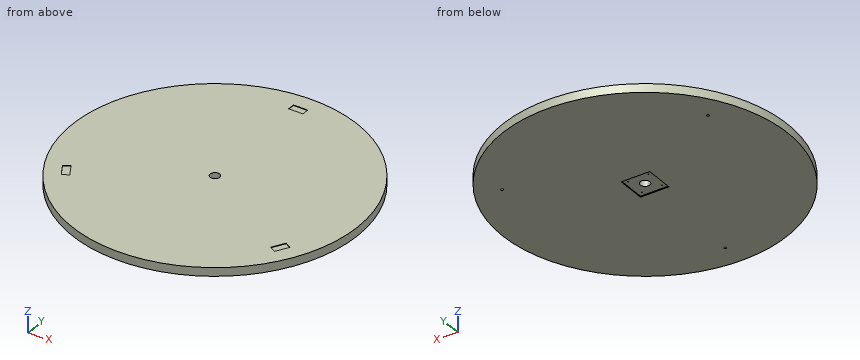
```python
from build123d import *

# Parameters (mm, degrees)
F0_R            = 300
F0_R_2          = 10
F1_DEPTH        = 18
F2_R            = 2.5
F3_DEPTH        = 10
F3_COPIES_COUNT = 3
F4_W            = 60
F4_H            = 60
F5_DEPTH        = 2
F6_R            = 1
F7_DEPTH        = 5
F7_COPIES_COUNT = 4
F8_W            = 30
F8_H            = 15
F9_DEPTH        = 1
F9_COPIES_COUNT = 3


# Not quite as in the source:
# - a pattern or mirror of a feature is missing from the dataset's text; its kind, count and spacing are read off the source's solid


with BuildPart() as f1:
    # F0 (on Top) → F1 (new body)
    with BuildSketch(Plane.XY):
        Circle(F0_R)
        Circle(F0_R_2, mode=Mode.SUBTRACT)
    extrude(amount=F1_DEPTH)

    # F2 (on face) → F3 (cut)
    with BuildSketch(Plane(origin=(0, 0, 0), x_dir=(1, 0, 0), z_dir=(0, 0, -1))):
        with Locations((0, 250)):
            Circle(F2_R)
    f3 = extrude(amount=-F3_DEPTH, mode=Mode.SUBTRACT)

    # F3_copies: F3 ×3 about axis
    f3_copies_axis = Axis((0, 0, 0), (0, 0, 1))
    for i in range(1, F3_COPIES_COUNT):
        add(f3.rotate(f3_copies_axis, i * 360 / F3_COPIES_COUNT), mode=Mode.SUBTRACT)

    # F4 (on face) → F5 (cut)
    with BuildSketch(Plane(origin=(0, 0, 0), x_dir=(1, 0, 0), z_dir=(0, 0, -1))):
        Rectangle(F4_W, F4_H)
    extrude(amount=-F5_DEPTH, mode=Mode.SUBTRACT)

    # F6 (on face) → F7 (cut)
    with BuildSketch(Plane(origin=(0, 0, 2), x_dir=(1, 0, 0), z_dir=(0, 0, -1))):
        with Locations((21.2132034356, 21.2132034356)):
            Circle(F6_R)
    f7 = extrude(amount=-F7_DEPTH, mode=Mode.SUBTRACT)

    # F7_copies: F7 ×4 about axis
    f7_copies_axis = Axis((0, 0, 0), (0, 0, 1))
    for i in range(1, F7_COPIES_COUNT):
        add(f7.rotate(f7_copies_axis, i * 360 / F7_COPIES_COUNT), mode=Mode.SUBTRACT)

    # F8 (on face) → F9 (cut)
    with BuildSketch(Plane.XY.offset(18)):
        with Locations((0, 260)):
            Rectangle(F8_W, F8_H)
    f9 = extrude(amount=-F9_DEPTH, mode=Mode.SUBTRACT)

    # F9_copies: F9 ×3 about axis
    f9_copies_axis = Axis((0, 0, 0), (0, 0, 1))
    for i in range(1, F9_COPIES_COUNT):
        add(f9.rotate(f9_copies_axis, i * 360 / F9_COPIES_COUNT), mode=Mode.SUBTRACT)


solid = f1.part
```
The model under review builds one solid part; all positions refer to its coordinate system, in mm. Round coordinates to 2 decimals unless told otherwise and drop trailing zeros. Loops run counter-clockwise (first coordinate to the right, second up) from the corner with the lowest first, then second, coordinate; pieces in that order, holes last. Notation, with made-up numbers: (-2.75, 44.5) -> (25.25, 44.5) arc R23 ccw to (25.25, 72.5) -> close; hole circle Ø4 at (4, 61.5). An arc over 180 degrees is marked (long way). Answer in a Markdown table with one row per item.
1) Consider section C-C, the plane y = 231.5. Write out the cut boundary in (x, z).
Taken from the geometry:
| item | result |
|---|---|
| outline | (-190.81, 0) -> (190.81, 0) -> (190.81, 18) -> (-190.81, 18) -> close |
2) Consider section A-A, the plane y = 0. Write out the cut boundary in (x, z), plus the area to 3 significant figures.
Taken from the geometry:
| item | result |
|---|---|
| outline | (-300, 0) -> (-30, 0) -> (-30, 2) -> (-10, 2) -> (-10, 18) -> (-300, 18) -> close; (10, 2) -> (30, 2) -> (30, 0) -> (300, 0) -> (300, 18) -> (10, 18) -> close |
| area | 10,400 mm² |
3) Wall thickness on line 1 along Y through (x, z) = (0, 6.25); line 2 along Y through (x, z) = (13, 1.75); line 3 along Y through (x, z) = (205, 1.25): over which ranges is each line inside the solid? List them lowest first.
Taken from the geometry:
| item | result |
|---|---|
| line 1 | y = -300 to -252.5, -247.5 to -10, 10 to 300 |
| line 2 | y = -299.72 to -30, 30 to 299.72 |
| line 3 | y = -219.03 to 219.03 |
4) Consider section B-B, the plane y = 79. Write out the cut boundary in (x, z), plus the area to 3 significant figures.
Taken from the geometry:
| item | result |
|---|---|
| outline | (-289.41, 0) -> (289.41, 0) -> (289.41, 18) -> (-289.41, 18) -> close |
| area | 10,400 mm² |
5) For pin 1 Ø3 at (x, z) = (147.5, 10.5) entering from -Y; pin 2 Ø0.5 at (y, z) = (262, 17.5) entering from +X; pin 3 Ø2 at (x, y) = (-21.5, 21) entering from -Z, all flat-tipped, find the tip position at first contact; note any pin that passes through.
Taken from the geometry:
| item | result |
|---|---|
| pin 1 | stops at y = -262.08 |
| pin 2 | stops at x = 146.58 |
| pin 3 | stops at z = 2 |
